Here's the drawing with two shaded views (mm, measured from the low corner). I have some questions. Round coordinates to 2 decimals unless told otherwise and drop trailing zeros. Loops run counter-clockwise (first coordinate to the right, second up) from the corner with the lowest first, then second, coordinate; pieces in that order, holes last. Notation, with made-up numbers: M -8.5,11.25 L 21.5,11.25 A20 ccw 21.5,34.25 Z; hole C 50,3.25 d2. An arc over 180 degrees is marked long. Answer as a JSON object with one key per item and string values.
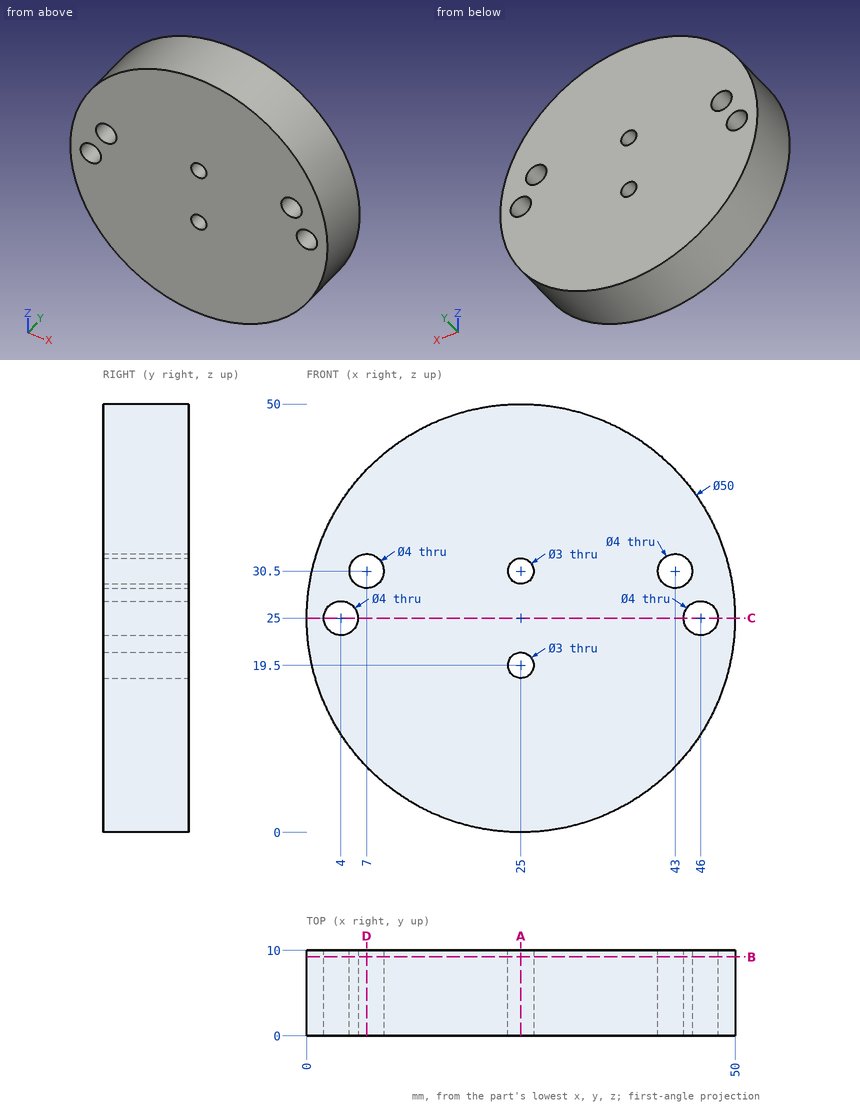
Item 1: I want a section at A-A on x = 25. List the corners of the cut face in (y, z) for me.
Solution:
{"outline": "M 0,0 L 10,0 L 10,18 L 0,18 Z; M 0,21 L 10,21 L 10,29 L 0,29 Z; M 0,32 L 10,32 L 10,50 L 0,50 Z"}
Item 2: If I drill on L1, parallel to Z at x = 25, y = 3.5; L2, parallel to X at y = 9.5, z = 30.5; L3, parallel to Z at x = 43, y = 7.25, over which ranges is the centre line in solid material (lowest first)? Write a range as from..to.
Solution:
{"L1": "z = 0..18, 21..29, 32..50", "L2": "x = 0.61..5, 9..23.5, 26.5..41, 45..49.39", "L3": "z = 7.65..28.5, 32.5..42.35"}
Item 3: I want a section at C-C on z = 25. List the corners of the cut face in (x, y) for me, plus the area to 3 significant figures.
Solution:
{"outline": "M 0,0 L 2,0 L 2,10 L 0,10 Z; M 6,0 L 44,0 L 44,10 L 6,10 Z; M 48,0 L 50,0 L 50,10 L 48,10 Z", "area": "420 mm2"}
Item 4: I want a section at B-B on y = 9.25. List the corners of the cut face in (x, z) for me, plus the area to 3 significant figures.
Solution:
{"outline": "C 25,25 d50; hole C 4,25 d4; hole C 7,30.5 d4; hole C 25,19.5 d3; hole C 25,30.5 d3; hole C 43,30.5 d4; hole C 46,25 d4", "area": "1,900 mm2"}
Item 5: For P1, Ø3, axis at y = 4.5, z = 30.5, coming from the -X side; P2, Ø2, axis at y = 4.5, z = 37, coming from the +X side, each with a flat end and sliding along its axis, tell me the tip position at first contact or that it passes through.
Solution:
{"P1": "stops at x = 0.32", "P2": "stops at x = 47.45"}
Item 6: I want a section at D-D on x = 7. List the corners of the cut face in (y, z) for me.
Solution:
{"outline": "M 0,7.65 L 10,7.65 L 10,28.5 L 0,28.5 Z; M 0,32.5 L 10,32.5 L 10,42.35 L 0,42.35 Z"}
